Work out the finished part from the listing and answer in its coordinate system (mm). Coordinates: 2 decimals unless noted, no trailing zeros. Write each loop counter-clockwise with the first axis right and the second up, starting at its lowest first coordinate (ties: lowest second). Pieces come first, ordered by that corner, then holes. Notation, with made-up numbers: (63.25, 75.5) - (112.25, 75.5) arc R30 cw to (112.25, 109.5) - close; hole circle Ø6 at (44.5, 30). An arc over 180 degrees is marked (long way). Use a Markdown table: item, result. Add a question column.
(1) Given pin 1 Ø6 at (y, z) = (25.5, 102) entering from +X; pin 2 Ø3 at (x, y) = (63, 12) entering from -Z; pin 3 Ø0.8 at (x, y) = (34, 10.5) entering from -Z, each flat-ended and moving along its own axis, determine where each tip first touches the part or whether it passes through.
(2) The part is cut by section C-C, the plane x = 75. Give the vertices of the cut face in (y, z).
(3) The part is cut by section A-A, the plane z = 146.05. Give the vertices of the cut face in (x, y) (3 decimals), then the cut area to 3 significant figures.
(4) The part is cut by section D-D, the plane y = 24. Give the vertices of the cut face in (x, z) (3 decimals).
(5) The part is cut by section B-B, the plane y = 12.5. Give the vertices of the cut face in (x, z) (3 decimals).
(6) Find the intervals of material crossed by line 1 (Z direction, x = 65, y = 19); line 2 (Y direction, x = 79, z = 42); line 3 (X direction, y = 9.5, z = 13), in increasing order. Write a range as from..to.
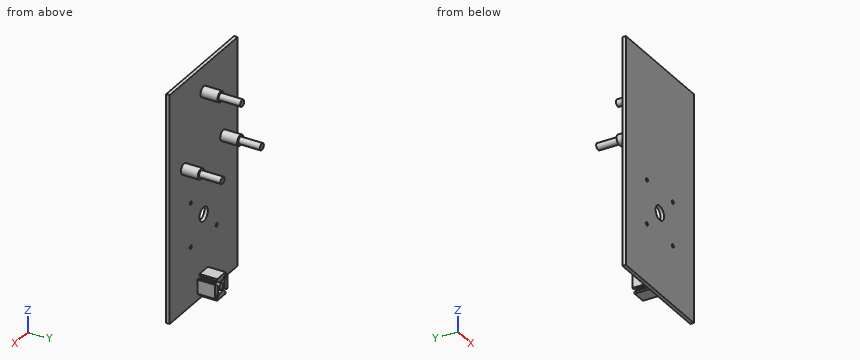
from build123d import *

# Parameters (mm, degrees)
SKETCH1_R               = 5.08
SKETCH1_R_2             = 1.27
BASE_EXTRUDE_DEPTH      = 2.54
SKETCH6_R               = 2.413
MIDDLE_BAR_HOLDER_DEPTH = 12.7
SKETCH7_R               = 2.413
BOSS_EXTRUDE6_DEPTH     = 27.686
SKETCH7_3_R             = 3.81
SKETCH7_3_R_2           = 2.413
BOSS_EXTRUDE7_DEPTH     = 12.192


with BuildPart() as part:
    # Sketch1 → base extrude (new body)
    with BuildSketch(Plane(origin=(0, 0, 0), x_dir=(1, 0, 0), z_dir=(0, 1, 0))):
        Polygon((82.55, -164.338), (82.55, -58.1000108), (82.55, 0), (0, 0), (0, -164.338), align=None)
        with Locations(Location((41.275, -58.1000108, 0), (0, 0, 270))):
            Circle(SKETCH1_R, mode=Mode.SUBTRACT)
        with Locations(Location((25.527, -42.3520108, 0), (0, 0, 270))):
            Circle(SKETCH1_R_2, mode=Mode.SUBTRACT)
        with Locations(Location((57.023, -42.3520108, 0), (0, 0, 270))):
            Circle(SKETCH1_R_2, mode=Mode.SUBTRACT)
        with Locations(Location((25.527, -73.8480108, 0), (0, 0, 270))):
            Circle(SKETCH1_R_2, mode=Mode.SUBTRACT)
        with Locations(Location((57.023, -73.8480108, 0), (0, 0, 270))):
            Circle(SKETCH1_R_2, mode=Mode.SUBTRACT)
    extrude(amount=BASE_EXTRUDE_DEPTH)

    # Sketch6 → middle bar holder (add)
    with BuildSketch(Plane(origin=(0, 2.54, 0), x_dir=(1, 0, 0), z_dir=(0, 1, 0))):
        Polygon((33.528, -9.906), (33.528, -4.826), (35.052, -4.826), (37.338, -7.366), (37.338, -9.906), (37.338, -12.446), (35.052, -14.986), (33.528, -14.986), align=None)
        with Locations(Location((41.275, -9.906, 0), (0, 0, 270))):
            Circle(SKETCH6_R)
        Polygon((41.275, -2.159), (46.355, -2.159), (46.355, -3.683), (43.815, -5.969), (41.275, -5.969), (38.735, -5.969), (36.195, -3.683), (36.195, -2.159), align=None)
        Polygon((47.498, -14.986), (45.212, -12.446), (45.212, -9.906), (45.212, -7.366), (47.498, -4.826), (49.022, -4.826), (49.022, -9.906), (49.022, -14.986), align=None)
        Polygon((41.275, -17.653), (36.195, -17.653), (36.195, -16.129), (38.735, -13.843), (41.275, -13.843), (43.815, -13.843), (46.355, -16.129), (46.355, -17.653), align=None)
    extrude(amount=MIDDLE_BAR_HOLDER_DEPTH)

    # Sketch7 → Boss-Extrude6 (add)
    with BuildSketch(Plane(origin=(0, 2.54, 0), x_dir=(1, 0, 0), z_dir=(0, 1, 0))):
        with Locations(Location((17.399, -102.616, 0), (0, 0, 270))):
            Circle(SKETCH7_R)
        with Locations(Location((41.275, -146.05, 0), (0, 0, 270))):
            Circle(SKETCH7_R)
        with Locations(Location((65.151, -102.616, 0), (0, 0, 270))):
            Circle(SKETCH7_R)
    extrude(amount=BOSS_EXTRUDE6_DEPTH)

    # Sketch7<3> → Boss-Extrude7 (add)
    # profile 1 of 3: a face of its own
    with BuildSketch(Plane(origin=(0, 2.54, 0), x_dir=(1, 0, 0), z_dir=(0, 1, 0))):
        with Locations(Location((41.275, -146.05, 0), (0, 0, 90))):
            Circle(SKETCH7_3_R)
        with Locations(Location((41.275, -146.05, 0), (0, 0, 270))):
            Circle(SKETCH7_3_R_2, mode=Mode.SUBTRACT)
    # profile 2 of 3: a face of its own
    with BuildSketch(Plane(origin=(0, 2.54, 0), x_dir=(1, 0, 0), z_dir=(0, 1, 0))):
        with Locations(Location((65.151, -102.616, 0), (0, 0, 90))):
            Circle(SKETCH7_3_R)
        with Locations(Location((65.151, -102.616, 0), (0, 0, 270))):
            Circle(SKETCH7_3_R_2, mode=Mode.SUBTRACT)
    # profile 3 of 3: a face of its own
    with BuildSketch(Plane(origin=(0, 2.54, 0), x_dir=(1, 0, 0), z_dir=(0, 1, 0))):
        with Locations(Location((17.399, -102.616, 0), (0, 0, 90))):
            Circle(SKETCH7_3_R)
        with Locations(Location((17.399, -102.616, 0), (0, 0, 270))):
            Circle(SKETCH7_3_R_2, mode=Mode.SUBTRACT)
    extrude(amount=BOSS_EXTRUDE7_DEPTH)


solid = part.part
Model answer:
| question | item | result |
|---|---|---|
| 1 | pin 1 | x = 67.56 |
| 1 | pin 2 | z = 98.86 |
| 1 | pin 3 | z = 4.83 |
| 2 | outline | (0, 0) - (2.54, 0) - (2.54, 164.34) - (0, 164.34) - close |
| 3 | outline | (0, 0) - (82.55, 0) - (82.55, 2.54) - (45.085, 2.54) - (45.085, 14.732) - (43.688, 14.732) - (43.688, 30.226) - (38.862, 30.226) - (38.862, 14.732) - (37.465, 14.732) - (37.465, 2.54) - (0, 2.54) - close |
| 3 | area | 377 mm^2 |
| 4 | outline | circle Ø4.826 at (17.399, 102.616); circle Ø4.826 at (41.275, 146.05); circle Ø4.826 at (65.151, 102.616) |
| 5 | outline | circle Ø7.62 at (17.399, 102.616); (33.528, 4.826) - (35.052, 4.826) - (37.338, 7.366) - (37.338, 12.446) - (35.052, 14.986) - (33.528, 14.986) - close; (36.195, 2.159) - (46.355, 2.159) - (46.355, 3.683) - (43.815, 5.969) - (38.735, 5.969) - (36.195, 3.683) - close; (36.195, 16.129) - (38.735, 13.843) - (43.815, 13.843) - (46.355, 16.129) - (46.355, 17.653) - (36.195, 17.653) - close; circle Ø7.62 at (41.275, 146.05); circle Ø4.826 at (41.275, 9.906); (45.212, 7.366) - (47.498, 4.826) - (49.022, 4.826) - (49.022, 14.986) - (47.498, 14.986) - (45.212, 12.446) - close; circle Ø7.62 at (65.151, 102.616) |
| 6 | line 1 | 100.21..105.02 |
| 6 | line 2 | 0..2.54 |
| 6 | line 3 | 33.53..36.84, 45.71..49.02 |
